Geometry check sheet. Reference: drawing and pictorial views, mm from the part's lowest x, y, z. Round coordinates to 2 decimals unless told otherwise and drop trailing zeros. Order: outer loops, then holes, each group sorted by start corner. A loop starts at its lowest first (then second) coordinate and runs counter-clockwise, first axis right, second up.
(1) Thickness scan on L1, parallel to Z at x = 0.3, y = 74; L2, parallel to Z at x = 0.5, y = 66; L3, parallel to Y at x = 2.25, z = 1.25 (3 decimals). Record the ranges inside material, lowest first.
(2) Cross-section at A-A on x = 2. Enter the section's corners in (y, z) (3 decimals), and give its area (3 significant figures).
(3) Cross-section at B-B on y = 7. Enter the section's corners in (x, z).
(4) Gauge pin test, flat ends, axial feed: P1, Ø0.9, axis at x = 2, z = 16.5, coming from the +Y side; P2, Ø1, axis at x = 1.5, y = 76, coming from the -Z side; P3, Ø1.5, axis at x = 1.5, z = 16, coming from the -Y side. Record the tip position at first contact, or that the pin passes through.
(5) Cross-section at C-C on y = 30. Enter the section's corners in (x, z).
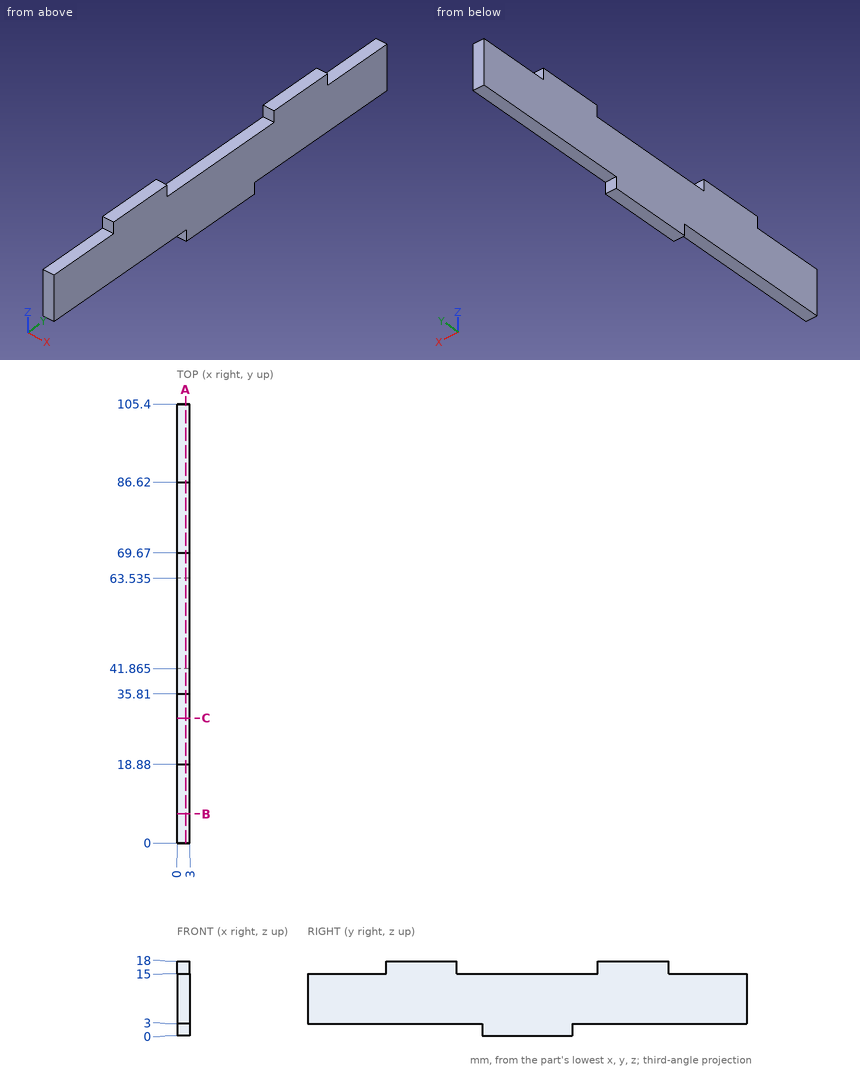
Found:
1. L1: z = 3 to 18
1. L2: z = 3 to 15
1. L3: y = 41.865 to 63.535
2. outline: (0, 3) - (41.865, 3) - (41.865, 0) - (63.535, 0) - (63.535, 3) - (105.4, 3) - (105.4, 15) - (86.62, 15) - (86.62, 18) - (69.67, 18) - (69.67, 15) - (35.81, 15) - (35.81, 18) - (18.88, 18) - (18.88, 15) - (0, 15) - close
2. area: 1,430 mm2
3. outline: (0, 3) - (3, 3) - (3, 15) - (0, 15) - close
4. P1: stops at y = 86.62
4. P2: stops at z = 3
4. P3: stops at y = 18.88
5. outline: (0, 3) - (3, 3) - (3, 18) - (0, 18) - close
